from build123d import *

# Parameters (mm, degrees)
SKETCH8_W           = 57.15
SKETCH8_H           = 127
BOSS_EXTRUDE3_DEPTH = 5.334
SKETCH9_R           = 16.505180298
CUT_EXTRUDE4_DEPTH  = 140.368483008
SKETCH12_W          = 19.05
SKETCH12_H          = 5.334
CUT_EXTRUDE8_DEPTH  = 5.334
SKETCH14_W          = 10.414
SKETCH14_H          = 5.334
BOSS_EXTRUDE4_DEPTH = 5.334
SKETCH15_W          = 5.207
SKETCH15_H          = 5.334
CUT_EXTRUDE9_DEPTH  = 5.334
SKETCH16_W          = 5.334
SKETCH16_H          = 4.5085
CUT_EXTRUDE10_DEPTH = 5.334
SKETCH19_W          = 4.7625
SKETCH19_H          = 4.5085
CUT_EXTRUDE12_DEPTH = 5.334
SKETCH20_W          = 5.334
SKETCH20_H          = 4.5085
CUT_EXTRUDE13_DEPTH = 145.225834933
SKETCH21_W          = 5.335765508
SKETCH21_H          = 0.4572
SKETCH21_W_2        = 5.334
SKETCH21_H_2        = 0.381
CUT_EXTRUDE14_DEPTH = 145.245837417


with BuildPart() as part:
    # Sketch8 → Boss-Extrude3 (new body)
    with BuildSketch(Plane.XY):
        with Locations((28.575, 63.5)):
            Rectangle(SKETCH8_W, SKETCH8_H)
    extrude(amount=BOSS_EXTRUDE3_DEPTH)

    # Sketch9 → Cut-Extrude4 (cut, through all)
    with BuildSketch(Plane.XY.offset(5.334)):
        with BuildLine():
            Line((46.736, 127), (10.414, 127))
            Line((10.414, 127), (12.069819702, 29.083))
            ThreePointArc((12.069819702, 29.083), (28.575, 45.588180298), (45.080180298, 29.083))
            Line((45.080180298, 29.083), (46.736, 127))
        make_face()
        with Locations((28.575, 29.083)):
            Circle(SKETCH9_R)
    extrude(amount=-CUT_EXTRUDE4_DEPTH, mode=Mode.SUBTRACT)

    # Sketch12 → Cut-Extrude8 (cut)
    with BuildSketch(Plane(origin=(0, 0, 0), x_dir=(-1, 0, 0), z_dir=(0, -1, 0))):
        with Locations((-47.625, -2.667)):
            Rectangle(SKETCH12_W, SKETCH12_H)
        with Locations((-9.525, -2.667)):
            Rectangle(SKETCH12_W, SKETCH12_H)
    extrude(amount=-CUT_EXTRUDE8_DEPTH, mode=Mode.SUBTRACT)

    # Sketch14 → Boss-Extrude4 (add)
    with BuildSketch(Plane(origin=(0, 127, 0), x_dir=(1, 0, 0), z_dir=(0, 1, 0))):
        with Locations((51.943, -2.667)):
            Rectangle(SKETCH14_W, SKETCH14_H)
        with Locations((5.207, -2.667)):
            Rectangle(SKETCH14_W, SKETCH14_H)
    extrude(amount=BOSS_EXTRUDE4_DEPTH)

    # Sketch15 → Cut-Extrude9 (cut)
    with BuildSketch(Plane(origin=(0, 132.334, 0), x_dir=(1, 0, 0), z_dir=(0, 1, 0))):
        with Locations((7.8105, -2.667)):
            Rectangle(SKETCH15_W, SKETCH15_H)
        with Locations((49.3395, -2.667)):
            Rectangle(SKETCH15_W, SKETCH15_H)
    extrude(amount=-CUT_EXTRUDE9_DEPTH, mode=Mode.SUBTRACT)

    # Sketch16 → Cut-Extrude10 (cut)
    with BuildSketch(Plane.ZY):
        with Locations((2.667, 7.58825)):
            Rectangle(SKETCH16_W, SKETCH16_H)
    extrude(amount=-CUT_EXTRUDE10_DEPTH, mode=Mode.SUBTRACT)

    # Sketch19 → Cut-Extrude12 (cut)
    with BuildSketch(Plane(origin=(57.15, 0, 0), x_dir=(0, 0, -1), z_dir=(1, 0, 0))):
        with Locations((-2.38125, 7.58825)):
            Rectangle(SKETCH19_W, SKETCH19_H)
    extrude(amount=-CUT_EXTRUDE12_DEPTH, mode=Mode.SUBTRACT)

    # Sketch20 → Cut-Extrude13 (cut, through all)
    with BuildSketch(Plane(origin=(0, 0, 4.7625), x_dir=(-1, 0, 0), z_dir=(0, 0, -1))):
        with Locations((-54.483, 7.58825)):
            Rectangle(SKETCH20_W, SKETCH20_H)
    extrude(amount=-CUT_EXTRUDE13_DEPTH, mode=Mode.SUBTRACT)

    # Sketch21 → Cut-Extrude14 (cut, through all)
    with BuildSketch(Plane.XY.offset(5.334)):
        with Locations((2.667882754, 10.0711)):
            Rectangle(SKETCH21_W, SKETCH21_H)
        with Locations((54.483, 10.033)):
            Rectangle(SKETCH21_W_2, SKETCH21_H_2)
    extrude(amount=-CUT_EXTRUDE14_DEPTH, mode=Mode.SUBTRACT)


solid = part.part
Input: part model. Units: mm. Frame: model coordinates. A direction names the side the tool comes from. Give positions to 0.01 mm unless a question says otherwise; leave off trailing zeros. Order: outer loops, then holes, each group sorted by start corner. A loop starts at its lowest first (then second) coordinate and runs counter-clockwise, first axis right, second up. Notation, with made-up numbers: (58, 69.25) - (73, 69.25) arc R21 cw to (73, 83.25) - close; hole circle Ø2 at (23, 55.25). An arc over 180 degrees is marked (long way). Answer as a JSON object with one key per item and string values. Group by question number.
Q1. Cut plane D-D, the plane y = 46.5. Output: boundary loops of the cut face in (x, z), then the cut area to 3 significant figures.
Q2. Cut plane A-A, the plane y = 14. Output: boundary loops of the cut face in (x, z).
Q3. Line query: probe 1 along Y at (x, z) = (5.5, 1.6); probe 2 along Y at (x, z) = (55.5, 0.7); probe 3 along X at (y, z) = (29, 5.05). Output: solid intervals per line, ascending.
Q4. First-contact query: pin 1 Ø2 at (x, z) = (18, 3.5) entering from -Y; pin 2 Ø1.5 at (x, z) = (26.5, 3.5) entering from -Y; pin 3 Ø1.6 at (x, z) = (54.5, 1.5) entering from -Y; pin 4 Ø1.6 at (x, z) = (3, 2.5) entering from -Y. Flat tips, straight axial feed; report the tip coordinate or a pass-through.
Q5. Mould query, pull axis X, two halves, no side actions, for faces 5 (the face through (38.1, 3, 3)), 6 (the face through (8, 127, 3)), 7 (the face through (3, 10.3, 3)). Classes: pulls with the +X half, pulls with the -X half, needs draft (parallel to the pull), parting line crosses it, or undercut.
Q6. Cut plane C-C, the plane x = 53.5. Output: boundary loops of the cut face in (y, z), then the cut area to 3 significant figures.
Q7. Set-up query: faces 1 (the face through (0, 70, 3)), 2 (the face through (54, 10.224, 3)), 3 (the face through (12, 5.334, 3)), 4 (the face through (5.207, 130, 3)). Return all of +Z, -Z, +X, -X, +Y, -Y with unobstructed straight access to the full face (end or side cutting, diameter ignored); none if empty.
Results:
{
 "1": {"outline": "(0, 0) - (11.78, 0) - (11.78, 5.33) - (0, 5.33) - close; (45.37, 0) - (57.15, 0) - (57.15, 5.33) - (45.37, 5.33) - close", "area": "126 mm^2"},
 "2": {"outline": "(0, 0) - (21.87, 0) - (21.87, 5.33) - (0, 5.33) - close; (35.28, 0) - (57.15, 0) - (57.15, 5.33) - (35.28, 5.33) - close"},
 "3": {"probe 1": "5.33 to 127", "probe 2": "10.22 to 132.33", "probe 3": "0 to 12.07, 45.08 to 57.15"},
 "4": {"pin 1": "y = 5.33", "pin 2": "y = 0", "pin 3": "y = 10.22", "pin 4": "y = 10.3"},
 "5": {"face 5": "pulls with the +X half", "face 6": "undercut", "face 7": "needs draft"},
 "6": {"outline": "(10.22, 0) - (132.33, 0) - (132.33, 5.33) - (10.22, 5.33) - close", "area": "651 mm^2"},
 "7": {"face 1": "+Z, -Z, -X, +Y, -Y", "face 2": "+Z, -Z, +X, -Y", "face 3": "+Z, -Z, -X, -Y", "face 4": "+Z, -Z, +Y"}
}
